Geometry check sheet. Reference: drawing and pictorial views, mm from the part's lowest x, y, z. A direction names the side the tool comes from. Coordinates: 2 decimals unless noted, no trailing zeros. Loops run counter-clockwise (first coordinate to the right, second up) from the corner with the lowest first, then second, coordinate; pieces in that order, holes last. Notation, with made-up numbers: (17.25, -36) -> (45.25, -36) arc R24 cw to (45.25, -22) -> close; hole circle Ø11 at (-11.75, 69.5). An arc over 180 degrees is marked (long way). Answer as a JSON object with one key per item and string values. Group by question number.
Q1. Gauge pin test, flat ends, axial feed: pin 1 Ø3 at (x, z) = (175.5, 8.5) entering from +Y; pin 2 Ø3.5 at (x, z) = (177, 7) entering from +Y; pin 3 Ø2 at (x, z) = (100, 1) entering from +Y. Record the tip position at first contact, or that the pin passes through.
Q2. Release check for a two-part mould opening along X. For the marked faces 3, 4 and 5 record: released by +X, released by -X, zero draft, split by the parting line, or undercut.
Q3. Cross-section at C-C on y = 19.25. Record the boundary of the cut face in (x, z).
Q4. Cross-section at B-B on z = 114. Record the boundary of the cut face in (x, y).
Q5. Cross-section at D-D on x = 168.27. Record the boundary of the cut face in (y, z).
Q6. Set-up check for the marked faces 1 and 2: record each of +Z, -Z, +X, -X, +Y, -Y from which the full face is reachable in a straight line by a thin tool's end or side.
Q7. Cross-section at A-A on x = 100.5. Record the boundary of the cut face in (y, z), and give its area (3 significant figures).
Q8. Scan lines: L1, parallel to Z at x = 7, y = 5.8; L2, parallel to X at y = 7.65, z = 7; L3, parallel to Z at x = 177, y = 7.1. Record each from-to range of solid material in increasing order.
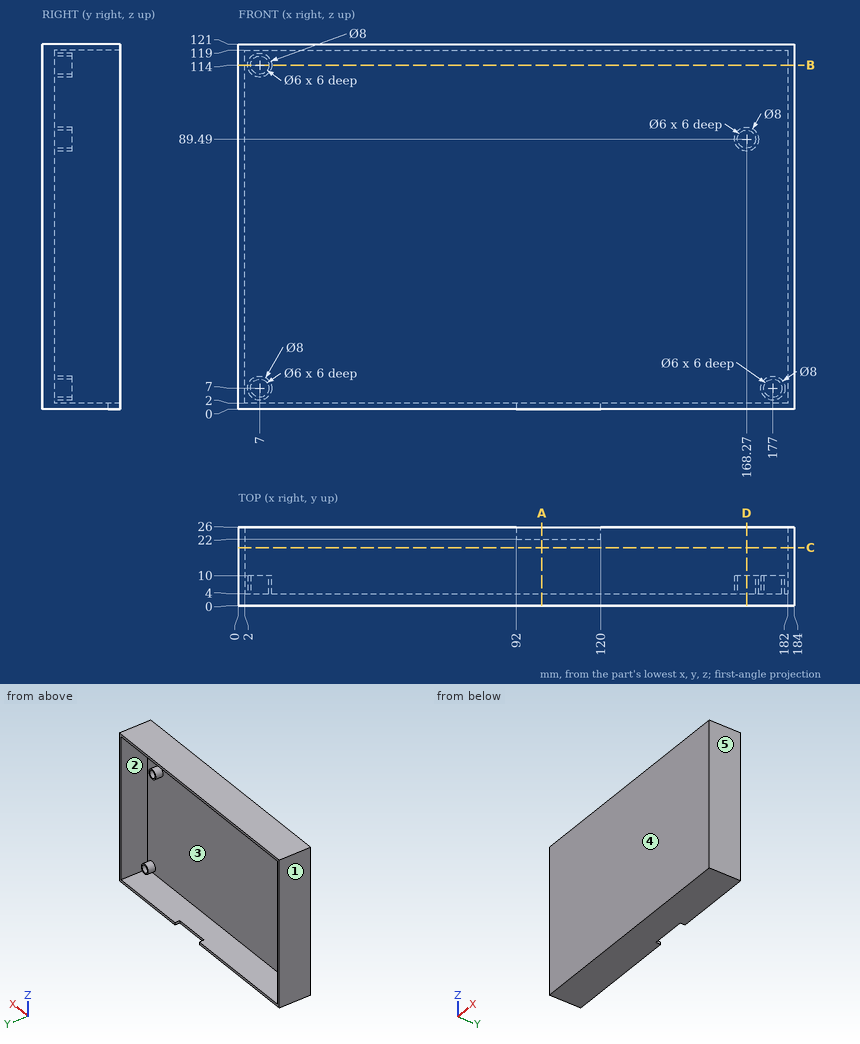
Computed values:
{
 "1": {"pin 1": "stops at y = 10", "pin 2": "stops at y = 4", "pin 3": "stops at y = 22"},
 "2": {"face 3": "undercut", "face 4": "zero draft", "face 5": "released by +X"},
 "3": {"outline": "(0, 0) -> (184, 0) -> (184, 121) -> (0, 121) -> close; hole (2, 2) -> (182, 2) -> (182, 119) -> (2, 119) -> close"},
 "4": {"outline": "(0, 0) -> (184, 0) -> (184, 26) -> (182, 26) -> (182, 4) -> (11, 4) -> (11, 10) -> (10, 10) -> (10, 4) -> (4, 4) -> (4, 10) -> (3, 10) -> (3, 4) -> (2, 4) -> (2, 26) -> (0, 26) -> close"},
 "5": {"outline": "(0, 0) -> (26, 0) -> (26, 2) -> (4, 2) -> (4, 85.49) -> (10, 85.49) -> (10, 86.49) -> (4, 86.49) -> (4, 92.49) -> (10, 92.49) -> (10, 93.49) -> (4, 93.49) -> (4, 119) -> (26, 119) -> (26, 121) -> (0, 121) -> close"},
 "6": {"face 1": "+Z, -Z, -X, +Y, -Y", "face 2": "+Y"},
 "7": {"outline": "(0, 0) -> (22, 0) -> (22, 2) -> (4, 2) -> (4, 119) -> (26, 119) -> (26, 121) -> (0, 121) -> close", "area": "564 mm²"},
 "8": {"L1": "z = 0 to 2, 3 to 4, 10 to 11, 110 to 111, 117 to 118, 119 to 121", "L2": "x = 0 to 2, 3 to 4, 10 to 11, 173 to 174, 180 to 181, 182 to 184", "L3": "z = 0 to 2, 3 to 4, 10 to 11, 119 to 121"}
}
